from build123d import *

# Parameters (mm, degrees)
F0_W     = 100
F0_H     = 30
F1_DEPTH = 10
F2_R     = 2
F2_R_2   = 5
F3_DEPTH = 25
F4_W     = 102.398372
F4_H     = 25
F5_DEPTH = 3
F6_R     = 14.995
F7_DEPTH = 10


with BuildPart() as f1:
    # F0 (on Front) → F1 (new body)
    with BuildSketch(Plane.XZ):
        Rectangle(F0_W, F0_H)
    extrude(amount=F1_DEPTH)

    # F2 (on face) → F3 (cut)
    with BuildSketch(Plane.XZ.offset(10)):
        with Locations((-32.5, 0)):
            Circle(F2_R)
        with Locations((32.5, 0)):
            Circle(F2_R)
        Circle(F2_R_2)
    extrude(amount=-F3_DEPTH, mode=Mode.SUBTRACT)

    # F4 (on face) → F5 (join)
    with BuildSketch(Plane.XY.offset(15)):
        with Locations((1.199186, 2.5)):
            Rectangle(F4_W, F4_H)
    extrude(amount=F5_DEPTH)

    # F6 (on face) → F7 (join)
    with BuildSketch(Plane(origin=(0, 0, 0), x_dir=(-1, 0, 0), z_dir=(0, 1, 0))):
        Circle(F6_R)
    extrude(amount=F7_DEPTH)


solid = f1.part
Geometry check sheet. Reference: the model listing, model coordinates, mm. A direction names the side the tool comes from. Round coordinates to 2 decimals unless told otherwise and drop trailing zeros. Write each loop counter-clockwise with the first axis right and the second up, starting at its lowest first coordinate (ties: lowest second). Pieces come first, ordered by that corner, then holes. Notation, with made-up numbers: (-23.5, 74.25) - (-18.5, 74.25) arc R27 cw to (-18.5, 100.25) - close; hole circle Ø8 at (50.5, -8.5). An arc over 180 degrees is marked (long way). One line per item, written item: value.
1. Cross-section at D-D on x = 0. Record the boundary of the cut face in (y, z) (3 decimals).
The answers:
outline: (-10, -15) - (0, -15) - (0, -14.995) - (10, -14.995) - (10, 14.995) - (0, 14.995) - (0, 15) - (15, 15) - (15, 18) - (-10, 18) - (-10, 5) - (0, 5) - (0, -5) - (-10, -5) - close
2. Depth check by flat-ended pin: pin 1 Ø10 at (x, z) = (16, 4) entering from +Y; pin 2 Ø4.5 at (x, z) = (-32.5, 0) entering from +Y; pin 3 Ø11 at (y, z) = (-3, -2.5) entering from +X; pin 4 Ø3 at (x, z) = (32.5, 0) entering from -Y. Enter the tip coordinate at first touch or a pass-through.
The answers:
pin 1: stops at y = 10
pin 2: stops at y = 0
pin 3: stops at x = 50
pin 4: passes through
3. Cross-section at A-A on x = 32.5. Record the boundary of the cut face in (y, z), and give its area (3 significant figures).
The answers:
outline: (-10, -15) - (0, -15) - (0, -2) - (-10, -2) - close; (-10, 2) - (0, 2) - (0, 15) - (15, 15) - (15, 18) - (-10, 18) - close
area: 335 mm^2
4. Cross-section at B-B on y = 9. Record the boundary of the cut face in (x, z) (3 decimals), and give its area (3 significant figures).
The answers:
outline: (-50, 15) - (52.398, 15) - (52.398, 18) - (-50, 18) - close; circle Ø29.99 at (0, 0)
area: 1,010 mm^2
5. Mould release check, pull along Z, two halves, no side actions. Record for faces 4 (the face through (50, -5, 0)), 5 (the face through (-1, -5, -15)), 6 (the face through (0, 3, 18)), 7 (the face through (-1.08, -5.07, -4.88)): released by +Z, released by -Z, zero draft, split by the parting line, or undercut.
The answers:
face 4: zero draft
face 5: released by -Z
face 6: released by +Z
face 7: undercut
6. Scan lines: L1, parallel to Z at x = -32.5, y = -6; L2, parallel to Y at x = -41, z = 6; L3, parallel to Z at x = -41.5, y = 4. Record each from-to range of solid material in increasing order.
The answers:
L1: z = -15 to -2, 2 to 18
L2: y = -10 to 0
L3: z = 15 to 18
7. Set-up check for faces 1 (the face through (0, 10, 0)), 2 (the face through (0, 0, 0)), 3 (the face through (52.398, 2, 16)): record each of +Z, -Z, +X, -X, +Y, -Y from which the full face is reachable in a straight line by a thin tool's end or side.
The answers:
face 1: -Z, +X, -X, +Y
face 2: -Y
face 3: +Z, -Z, +X, +Y, -Y
8. Cross-section at C-C on z = 0. Record the boundary of the cut face in (x, y) (3 decimals).
The answers:
outline: (-50, -10) - (-34.5, -10) - (-34.5, 0) - (-50, 0) - close; (-30.5, -10) - (-5, -10) - (-5, 0) - (5, 0) - (5, -10) - (30.5, -10) - (30.5, 0) - (14.995, 0) - (14.995, 10) - (-14.995, 10) - (-14.995, 0) - (-30.5, 0) - close; (34.5, -10) - (50, -10) - (50, 0) - (34.5, 0) - close
